Build history of the part. All positions in model axes, mm. Face numbers are marked on the shaded views. A direction names the side the tool comes from. Give positions to 0.01 mm unless a question says otherwise; leave off trailing zeros. Write each loop counter-clockwise with the first axis right and the second up, starting at its lowest first coordinate (ties: lowest second). Pieces come first, ordered by that corner, then holes.
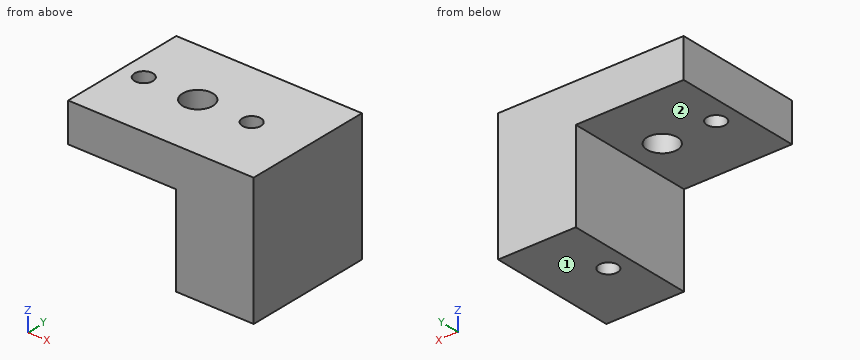
from build123d import *

# Parameters (mm, degrees)
SKETCH1_W           = 43
SKETCH1_H           = 30
SKETCH1_R           = 2.15
SKETCH1_R_2         = 3.5
BOSS_EXTRUDE1_DEPTH = 9
SKETCH2_W           = 18
SKETCH2_H           = 30
BOSS_EXTRUDE2_DEPTH = 21
SKETCH3_R           = 2.15
CUT_EXTRUDE1_DEPTH  = 340.846521731


with BuildPart() as part:
    # Sketch1 → Boss-Extrude1 (new body)
    with BuildSketch(Plane.XY):
        with Locations((-311.200177837, -47.5)):
            Rectangle(SKETCH1_W, SKETCH1_H)
        with Locations((-327.700177837, -47.5)):
            Circle(SKETCH1_R, mode=Mode.SUBTRACT)
        with Locations((-315.200177837, -47.5)):
            Circle(SKETCH1_R_2, mode=Mode.SUBTRACT)
    extrude(amount=BOSS_EXTRUDE1_DEPTH)

    # Sketch2 → Boss-Extrude2 (add)
    with BuildSketch(Plane(origin=(0, 0, 0), x_dir=(-1, 0, 0), z_dir=(0, 0, -1))):
        with Locations((298.700177837, -47.5)):
            Rectangle(SKETCH2_W, SKETCH2_H)
    extrude(amount=BOSS_EXTRUDE2_DEPTH)

    # Sketch3 → Cut-Extrude1 (cut, through all)
    with BuildSketch(Plane.XY.offset(9)):
        with Locations((-302.700177837, -47.5)):
            Circle(SKETCH3_R)
    extrude(amount=-CUT_EXTRUDE1_DEPTH, mode=Mode.SUBTRACT)


solid = part.part
(1) Saw through at B-B, the plane z = 6.75. List the corners of the cut face in (x, y).
(2) Probe line 1 (Z direction, x = -308, y = -46.5); line 2 (X direction, y = -57.5, z = -18.5); line 3 (X direction, y = -48.75, z = -18.25). List the from-to ranges inside material, lowest first.
(3) 3-axis set-ups, long thin cutter, end or side, ignore diameter. For the marked faces 1 and 2: which of +Z, -Z, +X, -X, +Y, -Y reach the whole face in a straight line?
(4) Saw through at D-D, the plane z = -0.5. List the corners of the cut face in (x, y), plus the area to 3 significant figures.
(5) Drop flat-ended pins along their axis: pin 1 (1 mm diameter, centred on x = -318, y = -46, fed in from +Z); pin 2 (2.5 mm diameter, centred on x = -302.7, y = -47.5, fed in from -Z); pin 3 (8 mm diameter, centred on x = -318.5, y = -54.5, fed in from -Z); pin 4 (8 mm diameter, centred on y = -50, z = -13, fed in from -X). Give the stop position or say it passes through.
(6) Saw through at A-A, the plane y = -47.5. List the corners of the cut face in (x, z).
(7) Saw through at C-C, the plane x = -315. List the corners of the cut face in (y, z).
Computed values:
1. outline: (-332.7, -62.5) - (-289.7, -62.5) - (-289.7, -32.5) - (-332.7, -32.5) - close; hole circle Ø4.3 at (-327.7, -47.5); hole circle Ø7 at (-315.2, -47.5); hole circle Ø4.3 at (-302.7, -47.5)
2. line 1: z = 0 to 9
2. line 2: x = -307.7 to -289.7
2. line 3: x = -307.7 to -304.45, -300.95 to -289.7
3. face 1: -Z, +X, -X, +Y, -Y
3. face 2: -Z, -X, +Y, -Y
4. outline: (-307.7, -62.5) - (-289.7, -62.5) - (-289.7, -32.5) - (-307.7, -32.5) - close; hole circle Ø4.3 at (-302.7, -47.5)
4. area: 525 mm2
5. pin 1: stops at z = 9
5. pin 2: passes through
5. pin 3: stops at z = 0
5. pin 4: stops at x = -307.7
6. outline: (-332.7, 0) - (-329.85, 0) - (-329.85, 9) - (-332.7, 9) - close; (-325.55, 0) - (-318.7, 0) - (-318.7, 9) - (-325.55, 9) - close; (-311.7, 0) - (-307.7, 0) - (-307.7, -21) - (-304.85, -21) - (-304.85, 9) - (-311.7, 9) - close; (-300.55, -21) - (-289.7, -21) - (-289.7, 9) - (-300.55, 9) - close
7. outline: (-62.5, 0) - (-50.99, 0) - (-50.99, 9) - (-62.5, 9) - close; (-44.01, 0) - (-32.5, 0) - (-32.5, 9) - (-44.01, 9) - close
